```python
from build123d import *

# Parameters (mm, degrees)
ESQUISSE1_R        = 2.5
BOSS_EXTRU_1_DEPTH = 10
ESQUISSE2_R        = 10
BOSS_EXTRU_2_DEPTH = 86.6
CONG_1_R           = 7.216666667


with BuildPart() as part:
    # Esquisse1 → Boss.-Extru.1 (new, symmetric)
    with BuildSketch(Plane.XY):
        with BuildLine():
            Line((5, 10), (5, -10))
            ThreePointArc((5, -10), (0, -15), (-5, -10))
            Line((-5, -10), (-5, 10))
            ThreePointArc((-5, 10), (0, 15), (5, 10))
        make_face()
        with Locations((0, 10)):
            Circle(ESQUISSE1_R, mode=Mode.SUBTRACT)
        with Locations((0, -10)):
            Circle(ESQUISSE1_R, mode=Mode.SUBTRACT)
    extrude(amount=BOSS_EXTRU_1_DEPTH, both=True)

    # Esquisse2 → Boss.-Extru.2 (add)
    with BuildSketch(Plane(origin=(5, 0, 0), x_dir=(0, 0, -1), z_dir=(1, 0, 0))):
        with Locations((0, 10)):
            Circle(ESQUISSE2_R)
    extrude(amount=BOSS_EXTRU_2_DEPTH)

    # Congé1
    cong_1_edges = [part.edges().sort_by_distance(p)[0] for p in [
        (91.6, 10, 10),
    ]]
    fillet(cong_1_edges, radius=CONG_1_R)


solid = part.part
```
Part model, mm, in its own coordinate system. A direction names the side the tool comes from. Give positions to 0.01 mm unless a question says otherwise; leave off trailing zeros. Write each loop counter-clockwise with the first axis right and the second up, starting at its lowest first coordinate (ties: lowest second). Pieces come first, ordered by that corner, then holes. Notation, with made-up numbers: (-7, 6.5) -> (-1, 6.5) arc R12 cw to (-1, 29.5) -> close; hole circle Ø4 at (18.5, 47). An arc over 180 degrees is marked (long way). Put each result on its own line as item: value. Start each with the question number.
Item 1: Pull direction X, two halves, no side cores. Call faces 4 (the face through (0, 15, 0)), 5 (the face through (91.6, 10, 0)), 6 (the face through (-5, 0, 0)): pulls with the +X half, pulls with the -X half, needs draft (parallel to the pull), parting line crosses it, or undercut.
Item 2: Wall check: L1, parallel to Y at x = 0, z = -4.25; L2, parallel to Y at x = 48.5, z = 0.5; L3, parallel to X at y = -3, z = 7.25. Give the ranges that are in metal, low to high. Write a range as [from, to].
Item 3: Cut at A-A (z = 0). State how many separate pieces and enclosed holes the cut face has, then the cut area to 3 significant figures.
Item 4: Which spindle directions (+Z, -Z, +X, -X, +Y, -Y) get a long thin tool onto all of the face, cutting with end or side? Do faces 1 (the face through (5, -4, 0)), 2 (the face through (0, 0, 10)), 3 (the face through (44.14, 0.24, 2.17)). Say none if no direction does.
Item 5: Pin check, flat tips, straight feed: pin 1 Ø6 at (x, y) = (31.5, 4) entering from +Z; pin 2 Ø10 at (x, y) = (56, 15.5) entering from +Z; pin 3 Ø12 at (x, z) = (39, 3.5) entering from -Y; pin 4 Ø4.5 at (x, y) = (0, -10) entering from +Z. Stop position of each tip, or through.
Item 6: Cut at C-C (x = 70). List the corners of the cut face in (y, z).
Answer list:
1. face 4: undercut
1. face 5: pulls with the +X half
1. face 6: pulls with the -X half
2. L1: y = [-15, -12.5], [-7.5, 7.5], [12.5, 15]
2. L2: y = [0.01, 19.99]
2. L3: x = [-5, 5]
3. separate pieces: 1
3. enclosed holes: 2
3. area: 1,950 mm2
4. face 1: +X, -Y
4. face 2: +Z, +X, -X, +Y, -Y
4. face 3: +X
5. pin 1: stops at z = 9.54
5. pin 2: stops at z = 9.99
5. pin 3: stops at y = 0
5. pin 4: passes through
6. outline: circle Ø20 at (10, 0)
